Autodesk Inventor part; units mm, degrees
ref_plane "YZ Plane" through (0, 0, 0) normal (1, 0, 0) x (0, 1, 0)
ref_plane "XZ Plane" through (0, 0, 0) normal (0, 1, 0) x (-1, 0, 0)
ref_plane "XY Plane" through (0, 0, 0) normal (0, 0, 1) x (1, 0, 0)
sketch "Sketch1" plane through (0, 0, 0) normal (0, 0, 1) x (1, 0, 0)
  line L0 (0, 0) -> (200, 0)
  line L1 (200, 0) -> (162.5, 150)
  line L2 (162.5, 150) -> (37.5, 150)
  line L3 (37.5, 150) -> (0, 0)
  dimension "d0" = 150
  dimension "d1" = 200
  dimension "d2" = 125
extrude "Extrusion1" add sketch "Sketch1" along normal blind 6.731
sketch "Sketch2" plane through (0, 0, 6.731) normal (0, 0, 1) x (1, 0, 0)
  line L0 (0, 0) -> (200, 0)
  line L1 (162.5, 150) -> (37.5, 150)
  line L2 (96.6345, 130) -> (103.3655, 130)
  line L3 (103.3655, 130) -> (103.3655, 100)
  line L4 (103.3655, 100) -> (96.6345, 100)
  line L5 (96.6345, 100) -> (96.6345, 130)
  point P0 (100, 130)
  point P1 (100, 150)
  dimension "d5" = 30
  dimension "d6" = 100
  dimension "d7" = 6.731
extrude "Extrusion2" cut sketch "Sketch2" against normal up to next
equation "\"d3\" = THICKB"
equation "\"d7\" = THICKB"
equation "\"THICKA\" = 3.175"
equation "\"THICKB\" = 6.731"
equation "\"THICKC\" = 12.7"
equation "\"THICKPLY\" = 5"
equation "\"MAGDIA\" = 9.5"
equation "\"BALLDIA\" = 12"
properties part number "Side"
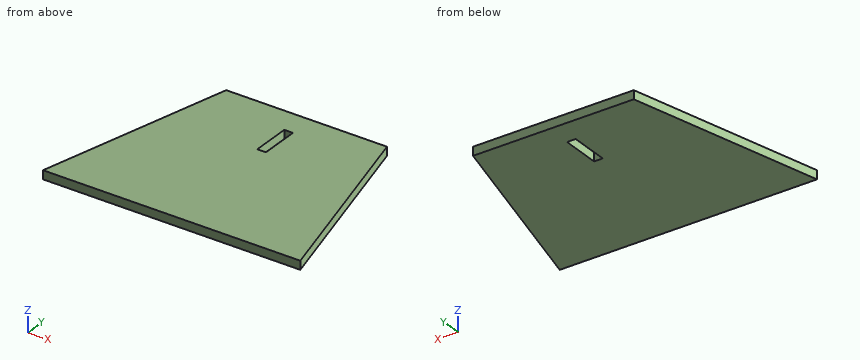
The listing builds one solid part. Answer for the finished solid, in the listing's coordinates (mm). Coordinates: 2 decimals unless noted, no trailing zeros. Loops run counter-clockwise (first coordinate to the right, second up) from the corner with the lowest first, then second, coordinate; pieces in that order, holes last. Notation, with made-up numbers: (67, 60.5) -> (115, 60.5) arc R12 ccw to (115, 82.5) -> close; hole circle Ø4 at (79, 21). An arc over 180 degrees is marked (long way). Use one line per item in the form item = value. Start each with the question number.
Item 1: The part is cut by section A-A on y = 121. Determine the outline of the cut face in (x, z), then the cut area to 3 significant figures.
Item 2: The part is cut by section D-D on y = 36. Determine the outline of the cut face in (x, z), then the cut area to 3 significant figures.
Item 3: Flat-ended cylindrical pins translate along their axes: pin 1 Ø3.5 at (x, z) = (99.5, 4) entering from -Y; pin 2 Ø4 at (y, z) = (36.5, 3.5) entering from +X (3 decimals); pin 3 Ø2 at (y, z) = (116.5, 4.5) entering from +X (3 decimals). Find the tip coordinate at first contact, or state that the pin passes through.
Item 4: Consider L1, parallel to Y at x = 97, z = 3.75; L2, parallel to X at y = 112.5, z = 3 (1 decimal); L3, parallel to X at y = 74.5, z = 5 (3 decimals). Determine where each line is inside the solid, lowest interval first. Write a range as [from, to].
Item 5: The part is cut by section C-C on x = 16. Determine the outline of the cut face in (y, z), then the cut area to 3 significant figures.
Item 6: The part is cut by section B-B on z = 1.5. Determine the outline of the cut face in (x, y), then the cut area to 3 significant figures.
Answer key:
q1.outline = (30.25, 0) -> (96.63, 0) -> (96.63, 6.73) -> (30.25, 6.73) -> close; (103.37, 0) -> (169.75, 0) -> (169.75, 6.73) -> (103.37, 6.73) -> close
q1.area = 894 mm2
q2.outline = (9, 0) -> (191, 0) -> (191, 6.73) -> (9, 6.73) -> close
q2.area = 1,230 mm2
q3.pin_1 = 0
q3.pin_2 = 191.375
q3.pin_3 = 171.125
q4.L1 = [0, 100], [130, 150]
q4.L2 = [28.1, 96.6], [103.4, 171.9]
q4.L3 = [18.625, 181.375]
q5.outline = (0, 0) -> (64, 0) -> (64, 6.73) -> (0, 6.73) -> close
q5.area = 431 mm2
q6.outline = (0, 0) -> (200, 0) -> (162.5, 150) -> (37.5, 150) -> close; hole (96.63, 100) -> (103.37, 100) -> (103.37, 130) -> (96.63, 130) -> close
q6.area = 24,200 mm2
